Geometry check sheet. Reference: the model listing, model coordinates, mm. A direction names the side the tool comes from. Give positions to 0.01 mm unless a question says otherwise; leave off trailing zeros. Write each loop counter-clockwise with the first axis right and the second up, starting at its lowest first coordinate (ties: lowest second). Pieces come first, ordered by that corner, then holes. Notation, with made-up numbers: (41, 20) -> (72, 20) arc R5 ccw to (72, 24) -> close; hole circle Ø7 at (85, -4). An arc over 180 degrees is marked (long way). Write item = value, one per line. Start each with the question number.
1. Cross-section at A-A, the plane z = 3.5. Record the cut outline in (x, y) (3 decimals).
2. Cross-section at D-D, the plane y = 13.25. State how many separate pieces and enclosed holes the cut face has, plus the area to 3 significant figures.
3. Mould release check, pull along Z, two halves, no side actions. Record for faces 6 (the flat face through (5, 13, 5.5)), 7 (the cylindrical face through (-6.705, 12.58, 2.523)), 8 (the cylindrical face through (-18.748, 12.733, 5.423)), 9 (the flat face through (18, 12, 0)): pulls with the +Z half, pulls with the -Z half, needs draft (parallel to the pull), parting line crosses it, or undercut.
4. Depth check by flat-ended pin: P1, Ø3, axis at x = 3.5, y = 11.5, coming from the +Z side; P2, Ø2, axis at x = -9, z = 4, coming from the +Y side; P3, Ø0.9, axis at x = 6, y = 13, coming from the -Z side; P4, Ø3, axis at y = 13.5, z = 7.5, coming from the +X side. Enter the tip coordinate at first touch or a pass-through.
5. Cross-section at B-B, the plane x = -15.25. Record the cut outline in (y, z), plus the area to 4 significant figures.
6. Cross-section at C-C, the plane y = 10.5. Record the cut outline in (x, z).
7. Thickness scan on line 1 along X through (y, z) = (13.5, 9.5); line 2 along X through (y, z) = (11.75, 10.25); line 3 along X through (y, z) = (11.25, 7). Record the ranges inside material, lowest first.
8. Set-up check for faces 1 (the flat face through (-3, 11.101, 4)), 2 (the flat face through (18, 12, 11)), 3 (the flat face through (-3, 14.101, 4)), 4 (the flat face through (5, 13, 2.75)), 5 (the cylindrical face through (0.44, 12.62, 6.18)): record each of +Z, -Z, +X, -X, +Y, -Y from which the full face is reachable in a straight line by a thin tool's end or side.
```python
from build123d import *

# Parameters (mm, degrees)
F1_DEPTH    = 11
F2_R        = 3.05
F3_DEPTH    = 3
F4_T1_DEPTH = 3
F4_T3_DEPTH = 17.7890113567
F5_R        = 5


# Not quite as in the source:
# - a fillet or chamfer that OpenCascade refuses, or shapes differently, is made with other operations: its cross-section is extruded or revolved along the edge and cut away or added


with BuildPart() as f1:
    # F0 (on Top) → F1 (new body)
    with BuildSketch(Plane.XY):
        with BuildLine():
            ThreePointArc((13.2813392877, 14.1006531194), (16.0415774558, 14.9456542135), (17.725, 12.6006531194))
            ThreePointArc((17.725, 12.6006531194), (16.0415774558, 10.2556520253), (13.2813392877, 11.1006531194))
            Line((13.2813392877, 11.1006531194), (12.0877223398, 11.1006531194))
            ThreePointArc((12.0877223398, 11.1006531194), (16.0187744108, 9.1861273975), (18.75, 12.6006531194))
            ThreePointArc((18.75, 12.6006531194), (16.0187744108, 16.0151788413), (12.0877223398, 14.1006531194))
            Line((12.0877223398, 14.1006531194), (13.2813392877, 14.1006531194))
        make_face()
        with BuildLine():
            ThreePointArc((13.2813392877, 11.1006531194), (12.775, 12.6006531194), (13.2813392877, 14.1006531194))
            Line((13.2813392877, 14.1006531194), (12.0877223398, 14.1006531194))
            ThreePointArc((12.0877223398, 14.1006531194), (11.75, 12.6006531194), (12.0877223398, 11.1006531194))
            Line((12.0877223398, 11.1006531194), (13.2813392877, 11.1006531194))
        make_face()
        with BuildLine():
            ThreePointArc((12.0877223398, 11.1006531194), (11.75, 12.6006531194), (12.0877223398, 14.1006531194))
            Line((12.0877223398, 14.1006531194), (-12.0877223398, 14.1006531194))
            ThreePointArc((-12.0877223398, 14.1006531194), (-11.8354742781, 13.3694275302), (-11.75, 12.6006531194))
            ThreePointArc((-11.75, 12.6006531194), (-11.8354742781, 11.8318787086), (-12.0877223398, 11.1006531194))
            Line((-12.0877223398, 11.1006531194), (12.0877223398, 11.1006531194))
        make_face()
        with BuildLine():
            ThreePointArc((-11.75, 12.6006531194), (-11.8354742781, 13.3694275302), (-12.0877223398, 14.1006531194))
            Line((-12.0877223398, 14.1006531194), (-13.2813392877, 14.1006531194))
            ThreePointArc((-13.2813392877, 14.1006531194), (-12.9049989059, 13.3922305752), (-12.775, 12.6006531194))
            ThreePointArc((-12.775, 12.6006531194), (-12.9049989059, 11.8090756636), (-13.2813392877, 11.1006531194))
            Line((-13.2813392877, 11.1006531194), (-12.0877223398, 11.1006531194))
            ThreePointArc((-12.0877223398, 11.1006531194), (-11.8354742781, 11.8318787086), (-11.75, 12.6006531194))
        make_face()
        with BuildLine():
            Line((-13.2813392877, 14.1006531194), (-12.0877223398, 14.1006531194))
            ThreePointArc((-12.0877223398, 14.1006531194), (-18.75, 12.6006531194), (-12.0877223398, 11.1006531194))
            Line((-12.0877223398, 11.1006531194), (-13.2813392877, 11.1006531194))
            ThreePointArc((-13.2813392877, 11.1006531194), (-17.725, 12.6006531194), (-13.2813392877, 14.1006531194))
        make_face()
    extrude(amount=F1_DEPTH)

    # F2 (on face) → F3 (cut, through all)
    with BuildSketch(Plane.XZ.offset(-11.1006531194)):
        with Locations((-6.0438611699, 5.5)):
            Circle(F2_R)
        Polygon((12.0877223398, 11), (-3.021930585, 11), (0, 5.5), (9.0657917549, 5.5), align=None)
        Polygon((10.5767570474, 2.75), (-1.5109652925, 2.75), (-3.021930585, 0), (12.0877223398, 0), align=None)
    extrude(amount=-F3_DEPTH, mode=Mode.SUBTRACT)

    # F4: fillet of radius 5 on 6 edges, made by hand

    # F4_s2 → F4_t1 (join)
    with BuildSketch(Plane.XZ.offset(-14.1006531194)):
        with BuildLine():
            ThreePointArc((2.9578022713, 5.5), (0.4120783796, 6.1965955492), (-1.4243095392, 8.0922840533))
            Line((-1.4243095392, 8.0922840533), (0, 5.5))
            Line((0, 5.5), (2.9578022713, 5.5))
        make_face()
        with BuildLine():
            ThreePointArc((10.4901012941, 8.0922840533), (8.6537133753, 6.1965955492), (6.1079894835, 5.5))
            Line((6.1079894835, 5.5), (9.0657917549, 5.5))
            Line((9.0657917549, 5.5), (10.4901012941, 8.0922840533))
        make_face()
    extrude(amount=F4_T1_DEPTH)

    # F4_s4 → F4_t3 (cut)
    with BuildSketch(Plane.XZ.offset(-21.4951587977)):
        with BuildLine():
            ThreePointArc((-1.5976210458, 8.4077159467), (-3.4340089645, 10.3034044508), (-5.9797328563, 11))
            Line((-5.9797328563, 11), (-3.021930585, 11))
            Line((-3.021930585, 11), (-1.5976210458, 8.4077159467))
        make_face()
        with BuildLine():
            ThreePointArc((-5.9797328563, 0), (-3.4340089645, 0.6965955492), (-1.5976210458, 2.5922840533))
            Line((-1.5976210458, 2.5922840533), (-3.021930585, 0))
            Line((-3.021930585, 0), (-5.9797328563, 0))
        make_face()
        with BuildLine():
            ThreePointArc((15.0455246112, 0), (12.4998007194, 0.6965955492), (10.6634128006, 2.5922840533))
            Line((10.6634128006, 2.5922840533), (12.0877223398, 0))
            Line((12.0877223398, 0), (15.0455246112, 0))
        make_face()
        with BuildLine():
            ThreePointArc((15.0455246112, 11), (12.4998007194, 10.3034044508), (10.6634128006, 8.4077159467))
            Line((10.6634128006, 8.4077159467), (12.0877223398, 11))
            Line((12.0877223398, 11), (15.0455246112, 11))
        make_face()
    extrude(amount=F4_T3_DEPTH, mode=Mode.SUBTRACT)

    # F5
    f5_edges = [f1.edges().sort_by_distance(p)[0] for p in [
        (10.576757, 12.600653, 2.75),
        (-1.510965, 12.600653, 2.75),
    ]]
    fillet(f5_edges, radius=F5_R)


solid = f1.part
```
Answers:
q1.outline = (-12.088, 11.101) -> (-8.347, 11.101) -> (-8.347, 14.101) -> (-12.088, 14.101) arc R3.5 ccw (long way) to start; (-3.741, 11.101) -> (12.088, 11.101) arc R3.5 ccw (long way) to (12.088, 14.101) -> (-3.741, 14.101) -> close; hole circle Ø4.95 at (-15.25, 12.601); hole circle Ø4.95 at (15.25, 12.601)
q2.separate_pieces = 3
q2.enclosed_holes = 1
q2.area = 172 mm^2
q3.face_6 = pulls with the +Z half
q3.face_7 = undercut
q3.face_8 = needs draft
q3.face_9 = pulls with the -Z half
q4.P1 = 5.59
q4.P2 = 14.1
q4.P3 = 2.75
q4.P4 = 18.75
q5.outline = (9.1, 0) -> (10.13, 0) -> (10.13, 11) -> (9.1, 11) -> close; (15.08, 0) -> (16.1, 0) -> (16.1, 11) -> (15.08, 11) -> close
q5.area = 22.55 mm^2
q6.outline = (-18.05, 0) -> (-16.56, 0) -> (-16.56, 11) -> (-18.05, 11) -> close; (-13.94, 0) -> (-12.45, 0) -> (-12.45, 11) -> (-13.94, 11) -> close; (12.45, 0.73) arc R5 ccw to (13.94, 0.12) -> (13.94, 10.88) arc R5 ccw to (12.45, 10.27) -> close; (16.56, 0) -> (18.05, 0) -> (18.05, 11) -> (16.56, 11) -> close
q7.line_1 = -18.63 to -17.56, -12.94 to -2.41, 11.47 to 12.94, 17.56 to 18.63
q7.line_2 = -18.65 to -17.57, -12.93 to -3.35, 12.41 to 12.93, 17.57 to 18.65
q7.line_3 = -18.48 to -17.32, -13.18 to -8.7, -3.39 to -0.61, 9.68 to 13.18, 17.32 to 18.48
q8.face_1 = +Z, -Z, -Y
q8.face_2 = +Z, +X, -X, +Y, -Y
q8.face_3 = +Z, -Z, +Y
q8.face_4 = -Z, +Y, -Y
q8.face_5 = +Z, +Y, -Y
